Check sheet for the modelled part. Datum: model origin and axes. Units: mm. Face numbers are marked on the shaded views. Give positions to 0.01 mm unless a question says otherwise; leave off trailing zeros. Order: outer loops, then holes, each group sorted by start corner. A loop starts at its lowest first (then second) coordinate and runs counter-clockwise, first axis right, second up. Notation, with made-up numbers: (8, -30) - (22, -30) arc R19 ccw to (22, -7) - close; hole circle Ø3 at (-28.5, 21). An arc over 180 degrees is marked (long way). Answer in a Markdown table with one row per item.
from build123d import *

# Parameters (mm, degrees)
SKETCH1_R           = 11.1125
SKETCH1_R_2         = 2.54
BOSS_EXTRUDE2_DEPTH = 5.08
FILLET1_R           = 7.62
CUT_EXTRUDE1_DEPTH  = 125.706848436
FILLET2_R           = 0.889


with BuildPart() as part:
    # Sketch1 → Boss-Extrude2 (new body)
    with BuildSketch(Plane(origin=(0, 0, 0), x_dir=(0, 0, -1), z_dir=(1, 0, 0))):
        Polygon((0, 0), (76.2, 0), (57.15, 99.798083649), (19.05, 99.798083649), align=None)
        with Locations((37.606341954, 74.398083649)):
            Circle(SKETCH1_R, mode=Mode.SUBTRACT)
        with Locations((37.606341954, 12.7)):
            Circle(SKETCH1_R_2, mode=Mode.SUBTRACT)
        with Locations((50.306341954, 12.7)):
            Circle(SKETCH1_R_2, mode=Mode.SUBTRACT)
        with Locations((63.006341954, 12.7)):
            Circle(SKETCH1_R_2, mode=Mode.SUBTRACT)
        with Locations((24.906341954, 12.7)):
            Circle(SKETCH1_R_2, mode=Mode.SUBTRACT)
        with Locations((12.206341954, 12.7)):
            Circle(SKETCH1_R_2, mode=Mode.SUBTRACT)
    extrude(amount=BOSS_EXTRUDE2_DEPTH)

    # Fillet1
    fillet1_edges = [part.edges().sort_by_distance(p)[0] for p in [
        (2.54, 99.798083649, -19.05),
        (2.54, 99.798083649, -57.15),
        (2.54, 0, -76.2),
        (2.54, 0, 0),
    ]]
    fillet(fillet1_edges, radius=FILLET1_R)

    # Sketch2 → Cut-Extrude1 (cut, through all)
    with BuildSketch(Plane(origin=(5.08, 0, 0), x_dir=(0, 0, -1), z_dir=(1, 0, 0))):
        Polygon((15.642904874, 62.107158672), (7.073205763, 17.452721053), (19.916541068, 40.570724603), align=None)
        Polygon((17.611424893, 62.107158672), (21.844949021, 40.570724603), (28.647489973, 40.570724603), (34.574296097, 62.107158672), align=None)
        Polygon((35.923336714, 62.107158672), (30.147133884, 40.570724603), (35.923336714, 17.219658997), align=None)
        Polygon((20.649761965, 39.113872964), (28.654674446, 39.113872964), (34.574296097, 17.219658997), (8.867656367, 17.219658997), align=None)
        Polygon((46.052866116, 40.570724603), (40.276663286, 17.219658997), (40.276663286, 62.107158672), align=None)
        Polygon((41.625703903, 17.219658997), (67.332343633, 17.219658997), (55.550238035, 39.113872964), (47.545325554, 39.113872964), align=None)
        Polygon((69.126794237, 17.452721053), (56.283458932, 40.570724603), (60.557095126, 62.107158672), align=None)
        Polygon((47.552510027, 40.570724603), (41.625703903, 62.107158672), (58.588575107, 62.107158672), (54.355050979, 40.570724603), align=None)
    extrude(amount=-CUT_EXTRUDE1_DEPTH, mode=Mode.SUBTRACT)

    # Fillet2
    fillet2_edges = [part.edges().sort_by_distance(p)[0] for p in [
        (2.54, 62.107158672, -17.611424893),
        (2.54, 62.107158672, -34.574296097),
        (2.54, 40.570724603, -28.647489973),
        (2.54, 40.570724603, -21.844949021),
        (2.54, 62.107158672, -35.923336714),
        (2.54, 17.219658997, -35.923336714),
        (2.54, 40.570724603, -30.147133884),
        (2.54, 40.570724603, -54.355050979),
        (2.54, 40.570724603, -47.552510027),
        (2.54, 62.107158672, -41.625703903),
        (2.54, 62.107158672, -58.588575107),
        (2.54, 17.219658997, -41.625703903),
        (2.54, 39.113872964, -47.545325554),
        (2.54, 39.113872964, -55.550238035),
        (2.54, 17.219658997, -67.332343633),
        (2.54, 62.107158672, -60.557095126),
        (2.54, 17.452721053, -69.126794237),
        (2.54, 40.570724603, -56.283458932),
        (2.54, 62.107158672, -15.642904874),
        (2.54, 40.570724603, -19.916541068),
        (2.54, 17.452721053, -7.073205763),
        (2.54, 62.107158672, -40.276663286),
        (2.54, 40.570724603, -46.052866116),
        (2.54, 17.219658997, -40.276663286),
        (2.54, 17.219658997, -34.574296097),
        (2.54, 17.219658997, -8.867656367),
        (2.54, 39.113872964, -20.649761965),
        (2.54, 39.113872964, -28.654674446),
    ]]
    fillet(fillet2_edges, radius=FILLET2_R)


solid = part.part
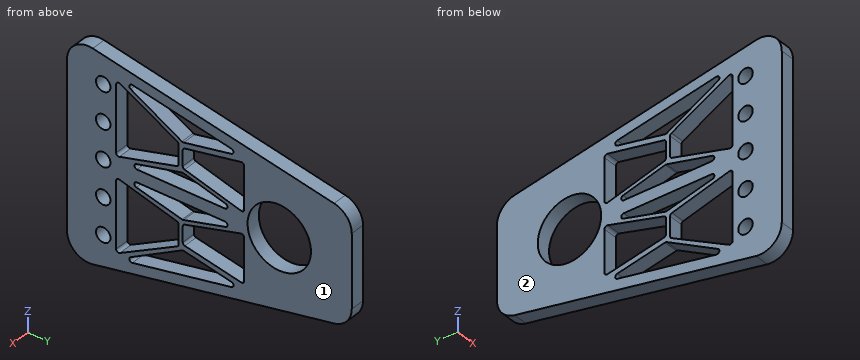
(1) Cross-section at B-B, the plane y = 12.7. Record the cut outline in (x, z), then the cut area to 3 significant figures.
Geometry says:
| item | result |
|---|---|
| outline | (0, -73.78) - (5.08, -73.78) - (5.08, -65.55) - (0, -65.55) - close; (0, -60.47) - (5.08, -60.47) - (5.08, -52.85) - (0, -52.85) - close; (0, -47.77) - (5.08, -47.77) - (5.08, -40.15) - (0, -40.15) - close; (0, -35.07) - (5.08, -35.07) - (5.08, -27.45) - (0, -27.45) - close; (0, -22.37) - (5.08, -22.37) - (5.08, -14.75) - (0, -14.75) - close; (0, -9.67) - (5.08, -9.67) - (5.08, -2.42) - (0, -2.42) - close |
| area | 233 mm² |
(2) Thickness scan on L1, parallel to Y at x = 3.8, z = -41; L2, parallel to Y at x = 2.5, z = -40.5; L3, parallel to Z at x = 3.1, y = 57.5. Record the ranges inside material, lowest first.
Geometry says:
| item | result |
|---|---|
| L1 | 0 to 23.64, 56.23 to 63.82, 84.98 to 99.8 |
| L2 | 0 to 23.93, 55.95 to 63.67, 85.13 to 99.8 |
| L3 | -65.22 to -61.44, -59.64 to -57.68, -42.89 to -33.31, -18.52 to -16.56, -14.76 to -10.98 |
(3) Cross-section at C-C, the plane y = 50. Record the cut outline in (x, z), then the cut area to 3 significant figures.
Geometry says:
| item | result |
|---|---|
| outline | (0, -66.66) - (5.08, -66.66) - (5.08, -62.88) - (0, -62.88) - close; (0, -58.15) - (5.08, -58.15) - (5.08, -56.21) - (0, -56.21) - close; (0, -44.96) - (5.08, -44.96) - (5.08, -43.52) - (0, -43.52) - close; (0, -40.28) - (5.08, -40.28) - (5.08, -35.92) - (0, -35.92) - close; (0, -32.68) - (5.08, -32.68) - (5.08, -31.24) - (0, -31.24) - close; (0, -19.99) - (5.08, -19.99) - (5.08, -18.05) - (0, -18.05) - close; (0, -13.32) - (5.08, -13.32) - (5.08, -9.54) - (0, -9.54) - close |
| area | 94.8 mm² |
(4) Mould release check, pull along X, two halves, no side actions. Record for the marked faces 1 and 2: pulls with the +X half, pulls with the -X half, needs draft (parallel to the pull), parting line crosses it, or undercut.
Geometry says:
| item | result |
|---|---|
| face 1 | pulls with the +X half |
| face 2 | pulls with the -X half |
(5) Gauge pin test, flat ends, axial feed: P1, Ø2.5, axis at x = 3.5, y = 45, coming from the -Z side; P2, Ø4, axis at y = 12.7, z = -37.61, coming from the +X side; P3, Ø2.5, axis at x = 3, y = 37, coming from the +Z side; P4, Ø2.5, axis at x = 1.5, z = -21, coming from the +Y side. Record the tip position at first contact, or that the pin passes through.
Geometry says:
| item | result |
|---|---|
| P1 | z = -67.85 |
| P2 | through |
| P3 | z = -6.82 |
| P4 | y = 99.14 |
(6) Cross-section at A-A, the plane z = -44. Record the cut outline in (x, y), then the cut area to 3 significant figures.
Geometry says:
| item | result |
|---|---|
| outline | (0, 0) - (5.08, 0) - (5.08, 17.22) - (0, 17.22) - close; (0, 26) - (5.08, 26) - (5.08, 32.27) - (0, 32.27) - close; (0, 48.22) - (5.08, 48.22) - (5.08, 53.48) - (0, 53.48) - close; (0, 62.11) - (5.08, 62.11) - (5.08, 65.31) - (0, 65.31) - close; (0, 83.49) - (5.08, 83.49) - (5.08, 99.8) - (0, 99.8) - close |
| area | 245 mm² |
(7) Cross-section at D-D, the plane x = 2.85. Give the number of separate pieces and of enclosed holes in the cut face, then the cut area to 3 significant figures.
Geometry says:
| item | result |
|---|---|
| separate pieces | 1 |
| enclosed holes | 14 |
| area | 3,310 mm² |
